The figure shows three views and two pictorial views of one solid part (mm, origin at its lowest corner). Answer the questions. Give positions to 0.01 mm unless a question says otherwise; leave off trailing zeros. Loops run counter-clockwise (first coordinate to the right, second up) from the corner with the lowest first, then second, coordinate; pieces in that order, holes last. Notation, with made-up numbers: (6, 45) - (25, 45) arc R31 ccw to (25, 73) - close; hole circle Ø7 at (46.5, 71.5). An arc over 180 degrees is marked (long way). Use CSV: the item, a comma, the result in double quotes.
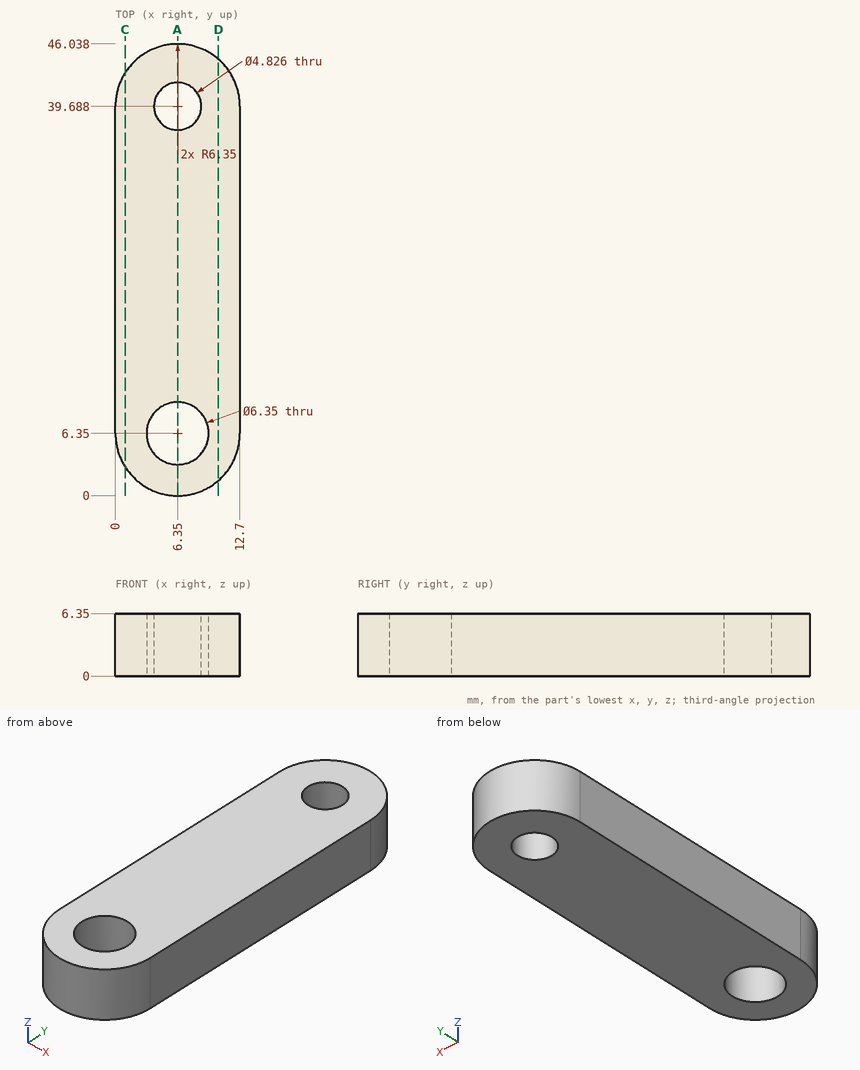
Item 1: Given P1, Ø3, axis at x = 5, y = 6, coming from the +Z side; P2, Ø2, axis at x = 2, z = 4.5, coming from the +Y side, each flat-ended and moving along its own axis, determine where each tip first touches the part or whether it passes through.
Determined:
P1,"passes through"
P2,"stops at y = 45.08"
Item 2: A cutting plane is placed at A-A on x = 6.35. State how many separate pieces and enclosed holes the cut face has, and give its area (3 significant figures).
Determined:
separate pieces,"3"
enclosed holes,"0"
area,"221 mm²"
Item 3: A cutting plane is placed at C-C on x = 1. Determine the outline of the cut face in (y, z), and give its area (3 significant figures).
Determined:
outline,"(2.93, 0) - (43.11, 0) - (43.11, 6.35) - (2.93, 6.35) - close"
area,"255 mm²"
Item 4: A cutting plane is placed at D-D on x = 10.5. Determine the outline of the cut face in (y, z), and give its area (3 significant figures).
Determined:
outline,"(1.54, 0) - (44.49, 0) - (44.49, 6.35) - (1.54, 6.35) - close"
area,"273 mm²"
Item 5: Find the intervals of material crossed by line 1 (Y direction, x = 6.35, z = 2.25) (1 decimal); line 2 (X direction, y = 9, z = 5); line 3 (Y direction, x = 3.75, z = 5.25) (1 decimal), in increasing order.
Determined:
line 1,"y = 0 to 3.2, 9.5 to 37.3, 42.1 to 46"
line 2,"x = 0 to 4.6, 8.1 to 12.7"
line 3,"y = 0.6 to 4.5, 8.2 to 45.5"
